Here's how the part is built. I have some questions about the finished solid (model axes, mm). Face numbers are marked on the shaded views. A direction names the side the tool comes from. Round coordinates to 2 decimals unless told otherwise and drop trailing zeros. Loops run counter-clockwise (first coordinate to the right, second up) from the corner with the lowest first, then second, coordinate; pieces in that order, holes last. Notation, with made-up numbers: M -25,-25.75 L 29,-25.75 A16 ccw 29,-21.75 Z; hole C 10,10.25 d9. An arc over 180 degrees is marked long. Use a Markdown table: item, result.
```python
from build123d import *

# Parameters (mm, degrees)
SKETCH2_W           = 1.754577672
SKETCH2_H           = 7.693148258
CUT_EXTRUDE1_DEPTH  = 10
SKETCH3_W           = 0.35
SKETCH3_H           = 2.35
BOSS_EXTRUDE1_DEPTH = 6
FILLET1_R           = 2


with BuildPart() as part:
    # Sketch1 → Revolve1 (revolve)
    with BuildSketch(Plane(origin=(0, 0, 0), x_dir=(1, 0, 0), z_dir=(0, 1, 0))):
        Polygon((-7.425, -2.233468586), (-5.75, -3.933468586), (0, -3.933468586), (0, 0), (0, 21.066531414), (-6, 21.066531414), (-6, -1.233468586), (-7.425, -1.233468586), align=None)
    revolve(axis=Axis((0, 0, -16.306049865), (0, 0, 1)))

    # Sketch2 → Cut-Extrude1 (cut)
    with BuildSketch(Plane.XY.offset(3.933468586)):
        Rectangle(SKETCH2_W, SKETCH2_H)
    extrude(amount=-CUT_EXTRUDE1_DEPTH, mode=Mode.SUBTRACT)

    # Sketch3 → Boss-Extrude1 (add)
    with BuildSketch(Plane(origin=(0, 0, -21.066531414), x_dir=(-1, 0, 0), z_dir=(0, 0, -1))):
        with Locations((-2.5, 0)):
            Rectangle(SKETCH3_W, SKETCH3_H)
        with Locations((2.5, 0)):
            Rectangle(SKETCH3_W, SKETCH3_H)
    extrude(amount=BOSS_EXTRUDE1_DEPTH)

    # Fillet1
    fillet1_edges = [part.edges().sort_by_distance(p)[0] for p in [
        (6, 0, -21.066531414),
    ]]
    fillet(fillet1_edges, radius=FILLET1_R)


solid = part.part
```
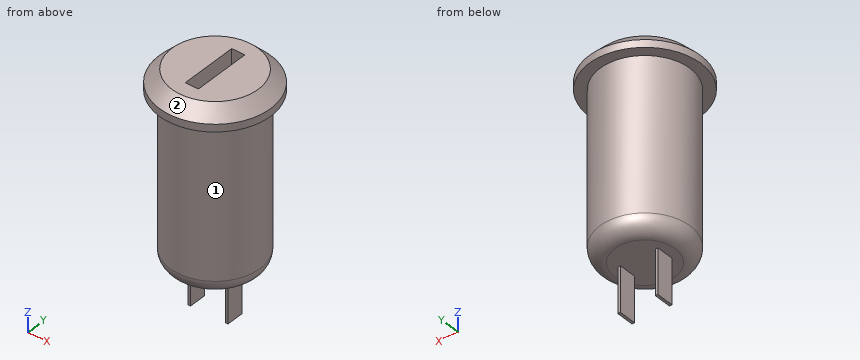
Q1. Imagine slicing it at B-B, the plane z = -4. Please give me the cut outline in (x, y), then the cut area to 3 significant figures.
Return value:
| item | result |
|---|---|
| outline | C 0,0 d12; hole M -0.88,-3.85 L 0.88,-3.85 L 0.88,3.85 L -0.88,3.85 Z |
| area | 99.6 mm^2 |
Q2. Imagine slicing it at C-C, the plane x = 0. Please give me the cut outline in (y, z) (3 decimals), then the cut area to 3 significant figures.
Return value:
| item | result |
|---|---|
| outline | M -7.425,1.233 L -6,1.233 L -6,-19.067 A2 ccw -4,-21.067 L 4,-21.067 A2 ccw 6,-19.067 L 6,1.233 L 7.425,1.233 L 7.425,2.233 L 5.75,3.933 L 3.847,3.933 L 3.847,-6.067 L -3.847,-6.067 L -3.847,3.933 L -5.75,3.933 L -7.425,2.233 Z |
| area | 226 mm^2 |
Q3. Will these pins go through, and if not, where does the flat tip stop? P1, Ø4.5, axis at x = 0.5, y = 3.5, coming from the -Z side; P2, Ø2, axis at x = -0.5, z = -12.5, coming from the -Y side; P3, Ø4, axis at y = -1.5, z = -2.5, coming from the -X side; P4, Ø5, axis at x = 2, y = 3.5, coming from the -Z side.
Return value:
| item | result |
|---|---|
| P1 | stops at z = -21.07 |
| P2 | stops at y = -6 |
| P3 | stops at x = -6 |
| P4 | stops at z = -27.07 |
Q4. For the marked faces 1 and 2, which set-ups out of +Z, -Z, +X, -X, +Y, -Y let a thin tool reach every point of the face, with its end or its side?
Return value:
| item | result |
|---|---|
| face 1 | -Z |
| face 2 | +Z |
Q5. Imagine slicing it at A-A, the plane y = 0. Please give me the cut outline in (x, z) (3 decimals).
Return value:
| item | result |
|---|---|
| outline | M -7.425,1.233 L -6,1.233 L -6,-19.067 A2 ccw -4,-21.067 L -2.675,-21.067 L -2.675,-27.067 L -2.325,-27.067 L -2.325,-21.067 L 2.325,-21.067 L 2.325,-27.067 L 2.675,-27.067 L 2.675,-21.067 L 4,-21.067 A2 ccw 6,-19.067 L 6,1.233 L 7.425,1.233 L 7.425,2.233 L 5.75,3.933 L 0.877,3.933 L 0.877,-6.067 L -0.877,-6.067 L -0.877,3.933 L -5.75,3.933 L -7.425,2.233 Z |
Q6. Imagine slicing it at D-D, the plane z = -14. Please give me the cut outline in (x, y).
Return value:
| item | result |
|---|---|
| outline | C 0,0 d12 |
Q7. I need wall thicknesses on line 1 (X direction, y = -0.75, z = -24.5) (3 decimals); line 2 (Y direction, x = 0.5, z = -0.5); line 3 (Z direction, x = -1.5, y = -2.25). Which ranges of each line are inside material? Lowest first, please. Write a range as from..to.
Return value:
| item | result |
|---|---|
| line 1 | x = -2.675..-2.325, 2.325..2.675 |
| line 2 | y = -5.98..-3.85, 3.85..5.98 |
| line 3 | z = -21.07..3.93 |
